Check sheet for the modelled part. Datum: model origin and axes. Units: mm. Face numbers are marked on the shaded views. Round coordinates to 2 decimals unless told otherwise and drop trailing zeros. Write each loop counter-clockwise with the first axis right and the second up, starting at its lowest first coordinate (ties: lowest second). Pieces come first, ordered by that corner, then holes. Notation, with made-up numbers: (33, -38) -> (70, -38) arc R8 cw to (70, -29) -> close; hole circle Ø4 at (13, -24). An arc over 180 degrees is marked (long way). One line per item, written item: value. Start each with the question number.
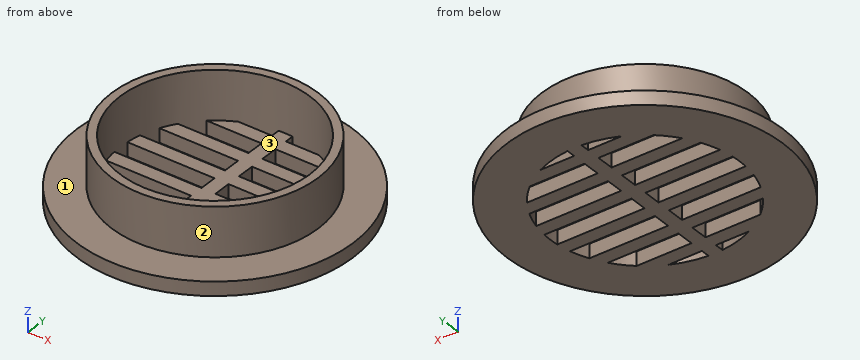
```python
from build123d import *

# Parameters (mm, degrees)
F0_R      = 19.75
F1_DEPTH  = 2
F3_W      = 29.5
F3_H      = 2
F4_DEPTH  = 2
F5_R      = 14.75
F6_DEPTH  = 2
F9_R      = 14.75
F9_R_2    = 13.55
F10_DEPTH = 9
F11_W     = 2
F11_H     = 33.5
F12_DEPTH = 2


with BuildPart() as f1:
    # F0 (on Top) → F1 (new body)
    with BuildSketch(Plane.XY):
        Circle(F0_R)
    extrude(amount=F1_DEPTH)


with BuildPart() as f4:
    # F3 (on face) → F4 (new body, through all)
    with BuildSketch(Plane.XY.offset(2)):
        with Locations((0, -15.75)):
            Rectangle(F3_W, F3_H)
    extrude(amount=-F4_DEPTH)


with BuildPart() as f4b:
    # F3 (on face) → F4, piece 2 (new body, through all)
    with BuildSketch(Plane.XY.offset(2)):
        with Locations((0, -11.25)):
            Rectangle(F3_W, F3_H)
    extrude(amount=-F4_DEPTH)


with BuildPart() as f4c:
    # F3 (on face) → F4, piece 3 (new body, through all)
    with BuildSketch(Plane.XY.offset(2)):
        with Locations((0, -6.75)):
            Rectangle(F3_W, F3_H)
    extrude(amount=-F4_DEPTH)


with BuildPart() as f4d:
    # F3 (on face) → F4, piece 4 (new body, through all)
    with BuildSketch(Plane.XY.offset(2)):
        with Locations((0, -2.25)):
            Rectangle(F3_W, F3_H)
    extrude(amount=-F4_DEPTH)


with BuildPart() as f4e:
    # F3 (on face) → F4, piece 5 (new body, through all)
    with BuildSketch(Plane.XY.offset(2)):
        with Locations((0, 2.25)):
            Rectangle(F3_W, F3_H)
    extrude(amount=-F4_DEPTH)


with BuildPart() as f4f:
    # F3 (on face) → F4, piece 6 (new body, through all)
    with BuildSketch(Plane.XY.offset(2)):
        with Locations((0, 6.75)):
            Rectangle(F3_W, F3_H)
    extrude(amount=-F4_DEPTH)


with BuildPart() as f4g:
    # F3 (on face) → F4, piece 7 (new body, through all)
    with BuildSketch(Plane.XY.offset(2)):
        with Locations((0, 11.25)):
            Rectangle(F3_W, F3_H)
    extrude(amount=-F4_DEPTH)


with BuildPart() as f4h:
    # F3 (on face) → F4, piece 8 (new body, through all)
    with BuildSketch(Plane.XY.offset(2)):
        with Locations((0, 15.75)):
            Rectangle(F3_W, F3_H)
    extrude(amount=-F4_DEPTH)


with BuildPart() as f6:
    # F5 (on Top) → F6 (new body, through all)
    with BuildSketch(Plane.XY):
        Circle(F5_R)
    extrude(amount=F6_DEPTH)

    # F7: cut F4h, F4g, F4f, F4e, F4d, F4c, F4b, F4
    add(f4h.part, mode=Mode.SUBTRACT)
    add(f4g.part, mode=Mode.SUBTRACT)
    add(f4f.part, mode=Mode.SUBTRACT)
    add(f4e.part, mode=Mode.SUBTRACT)
    add(f4d.part, mode=Mode.SUBTRACT)
    add(f4c.part, mode=Mode.SUBTRACT)
    add(f4b.part, mode=Mode.SUBTRACT)
    add(f4.part, mode=Mode.SUBTRACT)


with BuildPart() as f1_1:
    add(f1.part)

    # F8: cut F6
    add(f6.part, mode=Mode.SUBTRACT)

    # F9 (on face) → F10 (join, through all)
    with BuildSketch(Plane.XY):
        Circle(F9_R)
        Circle(F9_R_2, mode=Mode.SUBTRACT)
    extrude(amount=F10_DEPTH)

    # F11 (on face) → F12 (join, through all)
    with BuildSketch(Plane.XY):
        Rectangle(F11_W, F11_H)
    extrude(amount=F12_DEPTH)


solid = f1_1.part
```
1. Release check for a two-part mould opening along X. For the marked faces 1, 2 and 3 record: +X half, -X half, draft (parallel to the pull), parting line (faces both ways), or undercut.
2. Cross-section at A-A (y = 0). Record the cut outline in (x, z).
3. Cross-section at C-C (z = 6.75). Record the cut outline in (x, y), plus the area to 3 significant figures.
4. Material ranges on probe 1 along Y at (x, z) = (0, 3); probe 2 along Y at (x, z) = (7.5, 1.75); probe 3 along Z at (x, y) = (11, 12), recorded low to high.
5. Cross-section at B-B (x = 0). Record the cut outline in (y, z).
6. Cross-section at D-D (y = -4). Record the cut outline in (x, z).
7. Depth check by flat-ended pin: pin 1 Ø2 at (x, z) = (4, 1) entering from +Y; pin 2 Ø2 at (x, z) = (-9.5, 1) entering from +Y; pin 3 Ø2 at (x, z) = (-13, 5.5) entering from -Y. Enter the tip coordinate at first touch or a pass-through.
Working result:
1. face 1: draft
1. face 2: parting line
1. face 3: undercut
2. outline: (-19.75, 0) -> (-13.55, 0) -> (-13.55, 9) -> (-14.75, 9) -> (-14.75, 2) -> (-19.75, 2) -> close; (-1, 0) -> (1, 0) -> (1, 2) -> (-1, 2) -> close; (13.55, 0) -> (19.75, 0) -> (19.75, 2) -> (14.75, 2) -> (14.75, 9) -> (13.55, 9) -> close
3. outline: circle Ø29.5 at (0, 0); hole circle Ø27.1 at (0, 0)
3. area: 107 mm^2
4. probe 1: y = -14.75 to -13.55, 13.55 to 14.75
4. probe 2: y = -18.27 to -10.25, -7.75 to -5.75, -3.25 to -1.25, 1.25 to 3.25, 5.75 to 7.75, 10.25 to 18.27
4. probe 3: z = 0 to 2
5. outline: (-19.75, 0) -> (19.75, 0) -> (19.75, 2) -> (14.75, 2) -> (14.75, 9) -> (13.55, 9) -> (13.55, 2) -> (-13.55, 2) -> (-13.55, 9) -> (-14.75, 9) -> (-14.75, 2) -> (-19.75, 2) -> close
6. outline: (-19.34, 0) -> (-12.95, 0) -> (-12.95, 9) -> (-14.2, 9) -> (-14.2, 2) -> (-19.34, 2) -> close; (-1, 0) -> (1, 0) -> (1, 2) -> (-1, 2) -> close; (12.95, 0) -> (19.34, 0) -> (19.34, 2) -> (14.2, 2) -> (14.2, 9) -> (12.95, 9) -> close
7. pin 1: stops at y = 19.52
7. pin 2: stops at y = 17.83
7. pin 3: stops at y = -8.58
